Geometry check sheet. Reference: the model listing, model coordinates, mm. Face numbers are marked on the shaded views. A direction names the side the tool comes from. Round coordinates to 2 decimals unless told otherwise and drop trailing zeros. Write each loop counter-clockwise with the first axis right and the second up, starting at its lowest first coordinate (ties: lowest second). Pieces come first, ordered by that corner, then holes. Notation, with made-up numbers: M -5.5,5 L 11.5,5 A16 cw 11.5,31 Z; hole C -40,88.5 d11. An arc over 180 degrees is marked long. Answer as CSV lines item,"result". Start each with the question number.
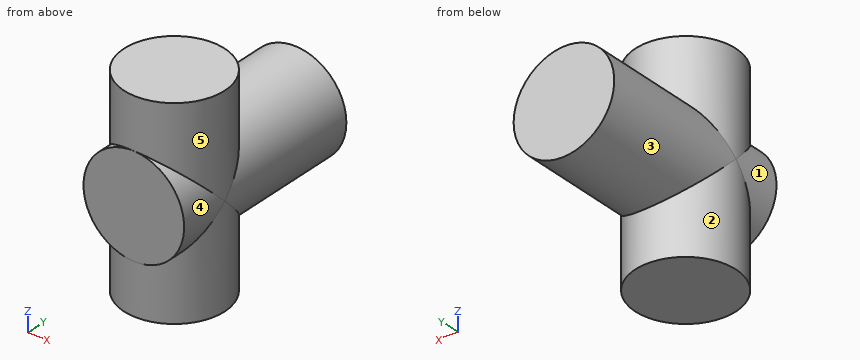
```python
from build123d import *

# Parameters (mm, degrees)
SKETCH1_R                = 25
BOSS_EXTRUDE1_DEPTH      = 100
SKETCH2_R                = 25
BOSS_EXTRUDE2_DEPTH      = 50
BOSS_EXTRUDE2_DEPTH_BACK = 50


with BuildPart() as part:
    # Sketch1 → Boss-Extrude1 (new body)
    with BuildSketch(Plane(origin=(0, 0, 0), x_dir=(1, 0, 0), z_dir=(0, 1, 0))):
        Circle(SKETCH1_R)
    extrude(amount=BOSS_EXTRUDE1_DEPTH)

    # Sketch2 → Boss-Extrude2 (add, two sides)
    with BuildSketch(Plane.XY) as boss_extrude2_sk:
        with Locations((0, 25)):
            Circle(SKETCH2_R)
    extrude(amount=BOSS_EXTRUDE2_DEPTH)
    extrude(boss_extrude2_sk.sketch, amount=-BOSS_EXTRUDE2_DEPTH_BACK)


solid = part.part
```
1) Section check A-A, the plane x = -15. Record the cut outline in (y, z).
2) Go/stop test with flat-tipped pins: pin 1 (1 mm diameter, centred on x = -10.5, z = -39.5, fed in from +Y); pin 2 (6 mm diameter, centred on x = 6, z = 31, fed in from -Y); pin 3 (3 mm diameter, centred on y = 19.5, z = 38.5, fed in from +X); pin 4 (5 mm diameter, centred on y = 27, z = -1, fed in from -X). Record where each tip stops, or that it passes through.
3) Scan lines: line 1 (Z direction, x = 0, y = 70); line 2 (X direction, y = 84, z = -12.5); line 3 (Y direction, x = -11.5, z = -24). Record each from-to range of solid material in increasing order. Write a range as from..to.
4) Section check B-B, the plane y = 10. Record the cut outline in (x, z).
5) Section check D-D, the plane z = -35.5. Record the cut outline in (x, y).
6) Access from +Z, -Z, +X, -X, +Y, -Y to the whole of each face (thin tool, end or side, straight path). Record for the marked faces 1, 2, 3, 4 and 5.
7) Section check C-C, the plane z = 17. Record the cut outline in (x, y), plus the area to 3 significant figures.
Results:
1,outline,"M 0,-20 L 5,-20 L 5,-50 L 45,-50 L 45,-20 L 100,-20 L 100,20 L 45,20 L 45,50 L 5,50 L 5,20 L 0,20 Z"
2,pin 1,"stops at y = 47.91"
2,pin 2,"stops at y = 0.18"
2,pin 3,"stops at x = 24.68"
2,pin 4,"stops at x = -25"
3,line 1,"z = -25..25"
3,line 2,"x = -21.65..21.65"
3,line 3,"y = 2.8..47.2"
4,outline,"M -20,-50 L 20,-50 L 20,-15 A25 ccw 20,15 L 20,50 L -20,50 L -20,15 A25 ccw -20,-15 Z"
5,outline,"C 0,25 d50"
6,face 1,"-X, -Y"
6,face 2,"-Z"
6,face 3,"+Y"
6,face 4,"+X, -Y"
6,face 5,"+Z"
7,outline,"M -18.33,0 L 18.33,0 L 18.33,8 A25 ccw 18.33,42 L 18.33,100 L -18.33,100 L -18.33,42 A25 ccw -18.33,8 Z"
7,area,"3,980 mm^2"
